from build123d import *

# Parameters (mm, degrees)
BASE_EXTRUDE_DEPTH = 12.7


with BuildPart() as part:
    # Sketch1 → Base-Extrude (new, symmetric)
    with BuildSketch(Plane.XY):
        with BuildLine():
            Line((-10.31875, 7.9375), (-10.31875, 1.016))
            ThreePointArc((-10.31875, 1.016), (-10.02117049, 0.29757951), (-9.30275, 0))
            Line((-9.30275, 0), (9.30275, 0))
            ThreePointArc((9.30275, 0), (10.02117049, 0.29757951), (10.31875, 1.016))
            Line((10.31875, 1.016), (10.31875, 7.9375))
            ThreePointArc((10.31875, 7.9375), (7.9375, 10.31875), (5.55625, 7.9375))
            Line((5.55625, 7.9375), (6.57225, 7.9375))
            ThreePointArc((6.57225, 7.9375), (7.9375, 9.30275), (9.30275, 7.9375))
            Line((9.30275, 7.9375), (9.30275, 1.016))
            Line((9.30275, 1.016), (-9.30275, 1.016))
            Line((-9.30275, 1.016), (-9.30275, 7.9375))
            ThreePointArc((-9.30275, 7.9375), (-7.9375, 9.30275), (-6.57225, 7.9375))
            Line((-6.57225, 7.9375), (-5.55625, 7.9375))
            ThreePointArc((-5.55625, 7.9375), (-7.9375, 10.31875), (-10.31875, 7.9375))
        make_face()
    base_extrude = extrude(amount=BASE_EXTRUDE_DEPTH, both=True)

    # Mirror1: Base-Extrude across plane
    add(base_extrude.mirror(Plane.ZX))


solid = part.part
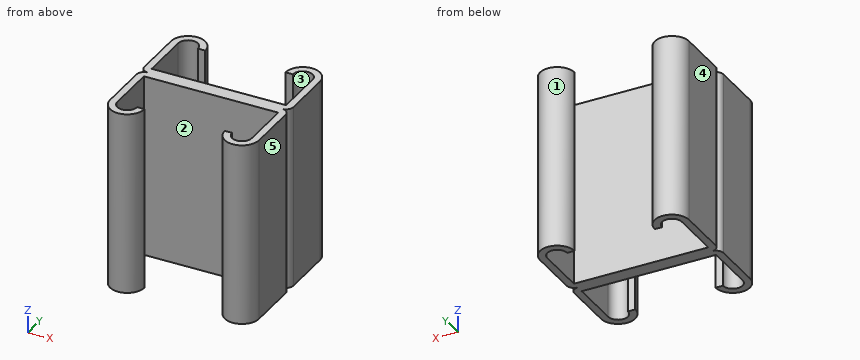
Read the model definition and answer for the solid it produces. Units are mm, in the model's axes. Face numbers are marked on the shaded views. A direction names the side the tool comes from. Round coordinates to 2 decimals unless told otherwise and drop trailing zeros. Order: outer loops, then holes, each group sorted by start corner. A loop starts at its lowest first (then second) coordinate and runs counter-clockwise, first axis right, second up. Notation, with made-up numbers: (-33.75, 50.25) - (-13.75, 50.25) arc R32 ccw to (-13.75, 85.25) - close; hole circle Ø10 at (16.5, 51.25). An arc over 180 degrees is marked (long way). Use one line per item in the form item = value. Start each with the question number.
(1) Flat-ended cylindrical pins translate along their axes: pin 1 Ø3 at (x, y) = (-2.5, 6.5) entering from +Z; pin 2 Ø3 at (x, z) = (5.5, 1) entering from -Y; pin 3 Ø1 at (x, z) = (-4, -0.5) entering from -Y; pin 4 Ø2 at (x, z) = (-3.5, 9) entering from +Y. Find the tip coordinate at first contact, or state that the pin passes through.
(2) The part is cut by section A-A (y = -2.5). Give the vertices of the cut face in (x, z).
(3) The part is cut by section C-C (x = -3.5). Give the vertices of the cut face in (y, z), then the cut area to 3 significant figures.
(4) Determine the mould class of the marked faces 3, 4 and 5 for opening direction X: +X half, -X half, draft (parallel to the pull), parting line (faces both ways), or undercut.
(5) The part is cut by section B-B (z = -10.25). Give the vertices of the cut face in (x, y), then the cut area to 3 significant figures.
(6) Find the intervals of material crossed by line 1 along Y through (x, z) = (8, -8); line 2 along X through (y, z) = (-6.5, 9.25); line 3 along Y through (x, z) = (-5.75, 5.75), in increasing order. Write a range as from..to.
(7) For the marked faces 1 and 2, determine the directions among +Z, -Z, +X, -X, +Y, -Y from which every point of the face is accessible in a straight line to the end or side of a thin tool.
Checked values:
q1.pin_1 = through
q1.pin_2 = -10.13
q1.pin_3 = -1.02
q1.pin_4 = 1.02
q2.outline = (-10.32, -12.7) - (-9.3, -12.7) - (-9.3, 12.7) - (-10.32, 12.7) - close; (9.3, -12.7) - (10.32, -12.7) - (10.32, 12.7) - (9.3, 12.7) - close
q3.outline = (-1.02, -12.7) - (1.02, -12.7) - (1.02, 12.7) - (-1.02, 12.7) - close
q3.area = 51.6 mm^2
q4.face_3 = undercut
q4.face_4 = -X half
q4.face_5 = +X half
q5.outline = (-10.32, -7.94) arc R2.38 ccw to (-5.56, -7.94) - (-6.57, -7.94) arc R1.37 cw to (-9.3, -7.94) - (-9.3, -1.02) - (9.3, -1.02) - (9.3, -7.94) arc R1.37 cw to (6.57, -7.94) - (5.56, -7.94) arc R2.38 ccw to (10.32, -7.94) - (10.32, -1.02) arc R1.02 ccw to (9.3, 0) arc R1.02 ccw to (10.32, 1.02) - (10.32, 7.94) arc R2.38 ccw to (5.56, 7.94) - (6.57, 7.94) arc R1.37 cw to (9.3, 7.94) - (9.3, 1.02) - (-9.3, 1.02) - (-9.3, 7.94) arc R1.37 cw to (-6.57, 7.94) - (-5.56, 7.94) arc R2.38 ccw to (-10.32, 7.94) - (-10.32, 1.02) arc R1.02 ccw to (-9.3, 0) arc R1.02 ccw to (-10.32, -1.02) - close
q5.area = 93.1 mm^2
q6.line_1 = -10.32..-9.3, -1.02..1.02, 9.3..10.32
q6.line_2 = -10.32..-9.3, 9.3..10.32
q6.line_3 = -8.88..-7.94, -1.02..1.02, 7.94..8.88
q7.face_1 = +Z, -Z, +Y
q7.face_2 = +Z, -Z
